Source: CAD feature listing. Evaluate the final solid. Frame: model axes, mm. A direction names the side the tool comes from. Give positions to 0.01 mm unless a question says otherwise; leave off trailing zeros. Loops run counter-clockwise (first coordinate to the right, second up) from the corner with the lowest first, then second, coordinate; pieces in that order, holes last. Notation, with made-up numbers: M -39.5,62.5 L -15.5,62.5 A11 ccw -15.5,72.5 Z; hole C 76.25,7 d11. An arc over 180 degrees is marked long. Put each result on its own line as item: value.
from build123d import *

# Parameters (mm, degrees)
F2_DEPTH = 40
F3_DEPTH = 10
F4_D     = 12
F5_D     = 11
F6_D     = 11


with BuildPart() as f2:
    # F0 (on Front) → F2 (new body)
    with BuildSketch(Plane.XZ):
        Polygon((-48, 10), (-48, 0), (-18, 0), (-18, 50), (18, 50), (18, 0), (48, 0), (48, 10), (28, 10), (28, 60), (-28, 60), (-28, 10), align=None)
    extrude(amount=F2_DEPTH)

    # F0 (on Front) → F3 (join)
    with BuildSketch(Plane.XZ):
        Polygon((48, 10), (28, 60), (28, 10), align=None)
        Polygon((-28, 60), (-48, 10), (-28, 10), align=None)
        Polygon((-18, 50), (-18, 0), (0, 0), (18, 0), (18, 50), align=None)
    extrude(amount=F3_DEPTH)

    # F4 (through all)
    with Locations(Plane(origin=(0, 0, 0), x_dir=(1, 0, 0), z_dir=(0, 0, -1))):
        with Locations((-4.172e-07, 25.0004983976)):
            Hole(F4_D / 2)

    # F5 (through all)
    with Locations(Plane(origin=(0, 0, 0), x_dir=(1, 0, 0), z_dir=(0, 0, -1))):
        with Locations((38.4999995828, 28.0004983976)):
            Hole(F5_D / 2)

    # F6 (through all)
    with Locations(Plane(origin=(0, 0, 0), x_dir=(1, 0, 0), z_dir=(0, 0, -1))):
        with Locations((-38.0000004172, 28.0004983976)):
            Hole(F6_D / 2)


solid = f2.part
1. Draft query along Y for faces 1 (the cylindrical face through (0.78, -30.95, 55.07)), 2 (the flat face through (0, -15, 60)), 3 (the flat face through (-1, 0, 30)), 4 (the flat face through (0, -10, 25)). Return one class per face: pulls with the +Y half, pulls with the -Y half, needs draft (parallel to the pull), parting line crosses it, or undercut.
Found:
face 1: undercut
face 2: needs draft
face 3: pulls with the +Y half
face 4: pulls with the -Y half
2. Contact query for flat-ended pins moving along their axis: P1, Ø16, axis at x = 34, z = 44, coming from the -Y side; P2, Ø15, axis at y = -29.5, z = 40.5, coming from the +X side; P3, Ø6, axis at x = 41.5, y = -27, coming from the +Z side; P4, Ø9, axis at x = 38.5, y = -28, coming from the +Z side. Output: stop coordinate, or through.
Found:
P1: y = -40
P2: x = 28
P3: z = 10
P4: through
3. Section query D-D (x = 13.5). Output: boundary loops of the cut face in (y, z), plus the area to 3 significant figures.
Found:
outline: M -40,50 L -10,50 L -10,0 L 0,0 L 0,60 L -40,60 Z
area: 900 mm^2
4. Material intervals for line 1 (X direction, y = -10.5, z = 24); line 2 (Y direction, x = 38.5, z = 8); line 3 (Z direction, x = -10, y = -17.5), sorted ascending. Write a range as from..to.
Found:
line 1: -28..-18, 18..28
line 2: -40..-33.5, -22.5..0
line 3: 50..60
5. Access query for faces 5 (the flat face through (-18, -25, 25)), 6 (the flat face through (-34, -10, 24)), 7 (the flat face through (48, -20, 5)), 8 (the flat face through (38, -21, 10)). Directions: +Z, -Z, +X, -X, +Y, -Y. A direction counts if a zero-diameter tool reaches every point of the face in a straight line with its end or side. Return the directions, or none.
Found:
face 5: -Z, -Y
face 6: +Z, -X, -Y
face 7: +Z, -Z, +X, +Y, -Y
face 8: +Z, +X, -Y
6. Section query B-B (z = 45.5). Output: boundary loops of the cut face in (x, y).
Found:
outline: M -33.8,-10 L -28,-10 L -28,-40 L -18,-40 L -18,-10 L 18,-10 L 18,-40 L 28,-40 L 28,-10 L 33.8,-10 L 33.8,0 L -33.8,0 Z
7. Section query A-A (x = 0). Output: boundary loops of the cut face in (y, z), plus the area to 3 significant figures.
Found:
outline: M -40,50 L -31,50 L -31,60 L -40,60 Z; M -19,50 L -10,50 L -10,0 L 0,0 L 0,60 L -19,60 Z
area: 780 mm^2
8. Section query C-C (y = -21.5). Output: boundary loops of the cut face in (x, z).
Found:
outline: M -48,0 L -18,0 L -18,50 L -4.87,50 L -4.87,60 L -28,60 L -28,10 L -48,10 Z; M 4.87,50 L 18,50 L 18,0 L 48,0 L 48,10 L 28,10 L 28,60 L 4.87,60 Z
